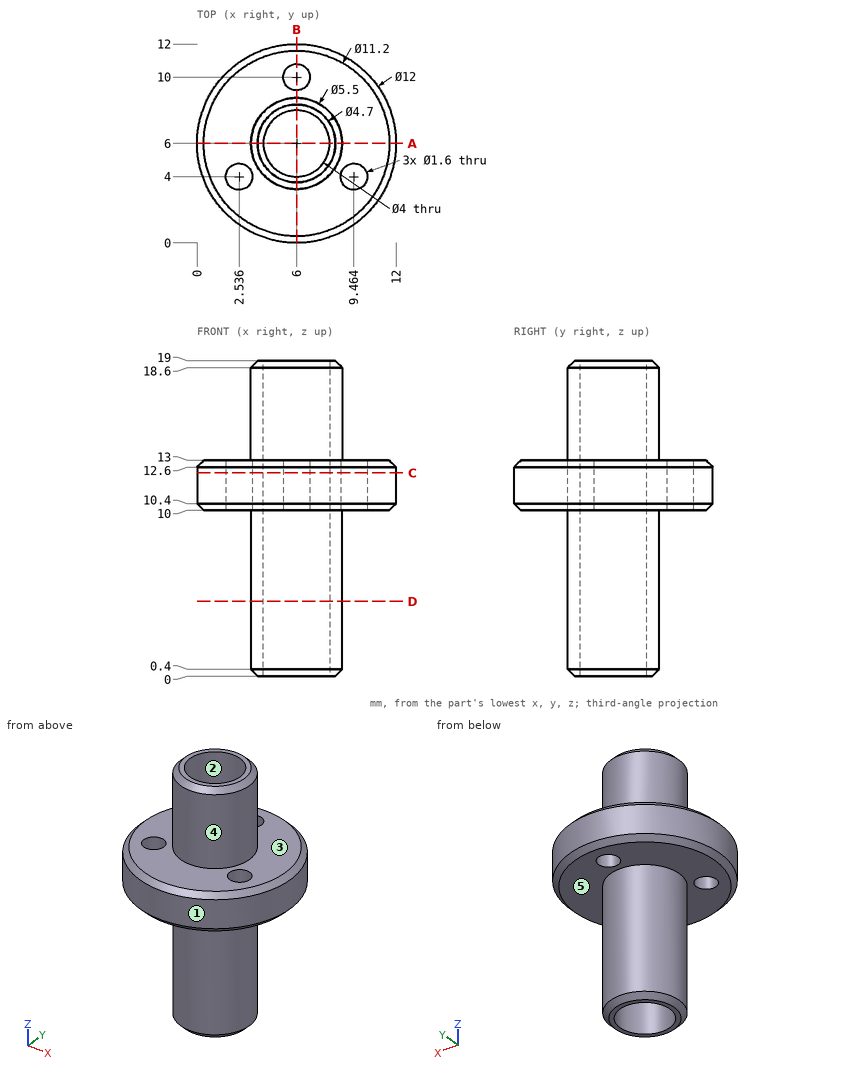
Here's the drawing with two shaded views (mm, measured from the low corner). I have some questions. A direction names the side the tool comes from. Give positions to 0.01 mm unless a question says otherwise; leave off trailing zeros. Loops run counter-clockwise (first coordinate to the right, second up) from the corner with the lowest first, then second, coordinate; pieces in that order, holes last. Notation, with made-up numbers: (66.5, -8.75) -> (111.5, -8.75) arc R21 ccw to (111.5, 14.25) -> close; hole circle Ø10 at (-4.5, 62.25). An arc over 180 degrees is marked (long way). Use one line per item in the form item = value.
1) If we section it at B-B (x = 6): Please give me the cut outline in (y, z).
Answers:
outline = (0, 10.4) -> (0.4, 10) -> (3.25, 10) -> (3.25, 0.4) -> (3.65, 0) -> (4, 0) -> (4, 19) -> (3.65, 19) -> (3.25, 18.6) -> (3.25, 13) -> (0.4, 13) -> (0, 12.6) -> close; (8, 0) -> (8.35, 0) -> (8.75, 0.4) -> (8.75, 10) -> (9.2, 10) -> (9.2, 13) -> (8.75, 13) -> (8.75, 18.6) -> (8.35, 19) -> (8, 19) -> close; (10.8, 10) -> (11.6, 10) -> (12, 10.4) -> (12, 12.6) -> (11.6, 13) -> (10.8, 13) -> close
2) Will these pins go through, and if not, where does the flat tip stop? pin 1 (6 mm diameter, centred on x = 6, z = 8.5, fed in from -Y); pin 2 (1.5 mm diameter, centred on x = 7.5, y = 2, fed in from -Z); pin 3 (1.4 mm diameter, centred on x = 9.46, y = 4, fed in from -Z); pin 4 (4 mm diameter, centred on x = 9, y = 10.5, fed in from +Z).
Answers:
pin_1 = 0
pin_2 = 10
pin_3 = through
pin_4 = 13
3) We'd pull the mould along Y, two halves only. Please class the marked faces 1, 2 and 3: released by +Y, released by -Y, zero draft, split by the parting line, or undercut.
Answers:
face_1 = split by the parting line
face_2 = undercut
face_3 = zero draft
4) I need wall thicknesses on line 1 along Y through (x, z) = (6, 11.4); line 2 along X through (y, z) = (4.5, 10.75); line 3 along Z through (x, y) = (11, 7.5). Which ranges of each line are inside material? Lowest first, please.
Answers:
line_1 = 0 to 4, 8 to 9.2, 10.8 to 12
line_2 = 0.19 to 1.91, 3.16 to 4.68, 7.32 to 8.84, 10.09 to 11.81
line_3 = 10 to 13
5) If we section it at A-A (y = 6): Please give me the cut outline in (x, z).
Answers:
outline = (0, 10.4) -> (0.4, 10) -> (3.25, 10) -> (3.25, 0.4) -> (3.65, 0) -> (4, 0) -> (4, 19) -> (3.65, 19) -> (3.25, 18.6) -> (3.25, 13) -> (0.4, 13) -> (0, 12.6) -> close; (8, 0) -> (8.35, 0) -> (8.75, 0.4) -> (8.75, 10) -> (11.6, 10) -> (12, 10.4) -> (12, 12.6) -> (11.6, 13) -> (8.75, 13) -> (8.75, 18.6) -> (8.35, 19) -> (8, 19) -> close
6) If we section it at C-C (z = 12.25): Please give me the cut outline in (x, y).
Answers:
outline = circle Ø12 at (6, 6); hole circle Ø1.6 at (2.54, 4); hole circle Ø4 at (6, 6); hole circle Ø1.6 at (6, 10); hole circle Ø1.6 at (9.46, 4)
7) If we section it at D-D (z = 4.5): Please give me the cut outline in (x, y), plus the area to 3 significant figures.
Answers:
outline = circle Ø5.5 at (6, 6); hole circle Ø4 at (6, 6)
area = 11.2 mm²
8) For the marked faces 4 and 5, which set-ups out of +Z, -Z, +X, -X, +Y, -Y let a thin tool reach every point of the face, with its end or its side?
Answers:
face_4 = +Z
face_5 = -Z
